```python
from build123d import *

# Parameters (mm, degrees)
SKETCH_1_W               = 55
SKETCH_1_H               = 35
EXTRUDE_1_DEPTH          = 16
SKETCH_3_R               = 2.65
CUT_EXTRUDE_2_DEPTH      = 13
SKETCH_4_W               = 12
SKETCH_4_H               = 12.75
CUT_EXTRUDE_3_DEPTH      = 68.126745787
FILLET_1_R               = 2
CUT_EXTRUDE_9_DEPTH      = 68.126745787
CUT_EXTRUDE_9_DEPTH_BACK = 18
SKETCH_11_R              = 1.4
SKETCH_12_W              = 6.8
SKETCH_12_H              = 16
CUT_EXTRUDE_10_DEPTH     = 68.126745787
SKETCH_13_W              = 15
SKETCH_13_H              = 15
SKETCH_13_W_2            = 20
CUT_EXTRUDE_12_DEPTH     = 13
SKETCH_15_W              = 20.5473163
SKETCH_15_H              = 18.952912532
CUT_EXTRUDE_13_DEPTH     = 13
SKETCH_16_W              = 5
SKETCH_16_H              = 16
CUT_EXTRUDE_14_DEPTH     = 12
FILLET_3_R               = 1


with BuildPart() as part:
    # 草图1 → 凸台-拉伸1 (new body)
    with BuildSketch(Plane.XY):
        with Locations((-27.5, 17.5)):
            Rectangle(SKETCH_1_W, SKETCH_1_H)
    extrude(amount=EXTRUDE_1_DEPTH)

    # 草图3 → 切除-拉伸2 (cut)
    with BuildSketch(Plane.XZ):
        with Locations(Location((-43, 8, 0), (0, 0, 270))):
            Circle(SKETCH_3_R)
        with Locations(Location((-7, 8, 0), (0, 0, 270))):
            Circle(SKETCH_3_R)
    extrude(amount=-CUT_EXTRUDE_2_DEPTH, mode=Mode.SUBTRACT)

    # 草图4 → 切除-拉伸3 (cut, through all)
    with BuildSketch(Plane.XZ):
        with Locations((-25, 6.375)):
            Rectangle(SKETCH_4_W, SKETCH_4_H)
    extrude(amount=-CUT_EXTRUDE_3_DEPTH, mode=Mode.SUBTRACT)

    # 圆角1
    fillet_1_edges = [part.edges().sort_by_distance(p)[0] for p in [
        (-55, 35, 8),
        (0, 35, 8),
        (0, 0, 8),
        (-55, 0, 8),
    ]]
    fillet(fillet_1_edges, radius=FILLET_1_R)

    # 草图11 → 切除-拉伸9 (cut, two sides: drawn at the far end of the back side and taken through both)
    with BuildSketch(Plane.ZY.offset(55).offset(-CUT_EXTRUDE_9_DEPTH_BACK)):
        with Locations(Location((12, 30, 0), (0, 0, 90))):
            Circle(SKETCH_11_R)
        with Locations(Location((2.5, 30, 0), (0, 0, 90))):
            Circle(SKETCH_11_R)
    extrude(amount=CUT_EXTRUDE_9_DEPTH + CUT_EXTRUDE_9_DEPTH_BACK, mode=Mode.SUBTRACT)

    # 草图12 → 切除-拉伸10 (cut, through all)
    with BuildSketch(Plane.XY.offset(16)):
        with Locations((-44.6, 27)):
            Rectangle(SKETCH_12_W, SKETCH_12_H)
    extrude(amount=-CUT_EXTRUDE_10_DEPTH, mode=Mode.SUBTRACT)

    # 草图13 → 切除-拉伸12 (cut)
    with BuildSketch(Plane.XY.offset(16)):
        with Locations((-7.5, 13.5)):
            Rectangle(SKETCH_13_W, SKETCH_13_H)
        with Locations((-45, 13.5)):
            Rectangle(SKETCH_13_W_2, SKETCH_13_H)
    extrude(amount=-CUT_EXTRUDE_12_DEPTH, mode=Mode.SUBTRACT)

    # 草图15 → 切除-拉伸13 (cut)
    with BuildSketch(Plane.XY.offset(16)):
        with Locations((-4.72634185, 30.476456266)):
            Rectangle(SKETCH_15_W, SKETCH_15_H)
    extrude(amount=-CUT_EXTRUDE_13_DEPTH, mode=Mode.SUBTRACT)

    # 草图16 → 切除-拉伸14 (cut)
    with BuildSketch(Plane(origin=(0, 35, 0), x_dir=(1, 0, 0), z_dir=(0, 1, 0))):
        with Locations((-35.7, -8)):
            Rectangle(SKETCH_16_W, SKETCH_16_H)
    extrude(amount=-CUT_EXTRUDE_14_DEPTH, mode=Mode.SUBTRACT)

    # 圆角3
    fillet_3_edges = [part.edges().sort_by_distance(p)[0] for p in [
        (-38.2, 23, 8),
        (-33.2, 23, 8),
        (-48, 19, 1.5),
        (-41.2, 19, 1.5),
    ]]
    fillet(fillet_3_edges, radius=FILLET_3_R)


solid = part.part
```
Can you work these out from the model? Positions are in its coordinate system, mm. A direction names the side the tool comes from. Give positions to 0.01 mm unless a question says otherwise; leave off trailing zeros. Loops run counter-clockwise (first coordinate to the right, second up) from the corner with the lowest first, then second, coordinate; pieces in that order, holes last. Notation, with made-up numbers: M 55,6 L 78,6 A28 ccw 78,40 Z; hole C 9.25,15 d2. An arc over 180 degrees is marked long. Use CSV: the item, a comma, the result in double quotes. Start each with the question number.
1. If we mould it in two halves opening along Y, with no side actions, what happens to faces 1 (the face through (-39.68, 28.6, 2.44)), 2 (the face through (-18, 35, 8)), 3 (the face through (-43, 14, 0))? For each: released by +Y, released by -Y, zero draft, split by the parting line, or undercut.
2. Imagine slicing it at D-D, the plane x = -36. Write out the boundary of the cut face in (y, z).
3. Imagine slicing it at C-C, the plane y = 30. Count the separate pieces of the cut face and the enclosed holes in it, plus the area to 3 significant figures.
4. If I drill on L1, parallel to Z at x = -53, y = 30; L2, parallel to X at y = 2.5, z = 8; L3, parallel to X at y = 31.5, z = 14, over which ranges is the centre line in solid material (lowest first)?
5. On a 3-axis mill with a long thin cutter (end or side, diameter ignored), from which of +Z, -Z, +X, -X, +Y, -Y can I reach the whole of each face in a straight line? I mean faces 4 (the face through (-40.37, 2.96, 8.34)), 5 (the face through (-39.68, 28.97, 11.05)), 6 (the face through (-19, 17, 6)), 7 (the face through (-48, 27, 8)). Say none if no direction works.
6. Imagine slicing it at B-B, the plane y = 25. Write out the boundary of the cut face in (x, z), plus the area to 3 significant figures.
7. For P1, Ø4, axis at x = -7, z = 8, coming from the -Y side; P2, Ø5.5, axis at y = 29.5, z = 6.5, coming from the +X side; P3, Ø1.5, axis at y = 13.5, z = 5, coming from the -X side; P4, Ø7.5, axis at x = -10.5, y = 24, coming from the +Z side, each with a flat end and sliding along its axis, tell me the tip position at first contact or that it passes through.
8. Imagine slicing it at A-A, the plane z = 14. Write out the boundary of the cut face in (x, y).
Response values:
1,face 1,"undercut"
1,face 2,"released by +Y"
1,face 3,"zero draft"
2,outline,"M 0,0 L 23,0 L 23,16 L 21,16 L 21,3 L 6,3 L 6,16 L 0,16 Z"
3,separate pieces,"7"
3,enclosed holes,"0"
3,area,"287 mm^2"
4,L1,"0 to 1.1, 3.9 to 10.6, 13.4 to 16"
4,L2,"-55 to -45.65, -40.35 to -31, -19 to -9.65, -4.35 to 0"
4,L3,"-55 to -48, -41.2 to -38.2, -33.2 to -15"
5,face 4,"-Y"
5,face 5,"-X"
5,face 6,"-Z, +Y, -Y"
5,face 7,"+Z, -Z, +Y"
6,outline,"M -55,0 L -48,0 L -48,16 L -55,16 Z; M -41.2,0 L -38.2,0 L -38.2,16 L -41.2,16 Z; M -33.2,0 L -31,0 L -31,12.75 L -19,12.75 L -19,0 L 0,0 L 0,3 L -15,3 L -15,16 L -33.2,16 Z"
6,area,"343 mm^2"
7,P1,"through"
7,P2,"x = -15"
7,P3,"x = -35"
7,P4,"z = 3"
8,outline,"M -55,2 A2 ccw -53,0 L -2,0 A2 ccw 0,2 L 0,6 L -15,6 L -15,35 L -33.2,35 L -33.2,24 A1 cw -34.2,23 L -37.2,23 A1 cw -38.2,24 L -38.2,35 L -41.2,35 L -41.2,21 L -35,21 L -35,6 L -55,6 Z; M -55,21 L -48,21 L -48,35 L -53,35 A2 ccw -55,33 Z"
